from build123d import *

# Parameters (mm, degrees)
F0_R      = 7.65
F0_R_2    = 4.65
F1_DEPTH  = 20
F4_DEPTH  = 20.001
F6_R      = 0.775
F7_DEPTH  = 1.0786128078
F9_R      = 0.775
F10_DEPTH = 1.0463142634
F12_R     = 0.775
F13_DEPTH = 1.0463142634
F14_W     = 1
F14_H     = 5.2947397344
F15_DEPTH = 20
F16_R     = 0.835
F17_DEPTH = 20
F18_W     = 3.1734104046
F18_H     = 10
F19_DEPTH = 15.2846427429


with BuildPart() as f1:
    # F0 (on Top) → F1 (new body)
    with BuildSketch(Plane.XY):
        Circle(F0_R)
        Circle(F0_R_2, mode=Mode.SUBTRACT)
    extrude(amount=F1_DEPTH)

    # F2 (on face) → F4 (cut, through all)
    with BuildSketch(Plane.XY.offset(20)):
        with BuildLine():
            Line((-3.4395020739, 4.4824463726), (-4.0482635029, 5.2757997129))
            ThreePointArc((-4.0482635029, 5.2757997129), (-5.7590689352, 3.325), (-6.5931083281, 0.8679991783))
            Line((-6.5931083281, 0.8679991783), (-5.6016634668, 0.737472986))
            ThreePointArc((-5.6016634668, 0.737472986), (-4.8930435314, 2.825), (-3.4395020739, 4.4824463726))
        make_face()
        with BuildLine():
            Line((4.0482635029, 5.2757997129), (3.4395020739, 4.4824463726))
            ThreePointArc((3.4395020739, 4.4824463726), (4.8930435314, 2.825), (5.6016634668, 0.737472986))
            Line((5.6016634668, 0.737472986), (6.5931083281, 0.8679991783))
            ThreePointArc((6.5931083281, 0.8679991783), (5.7590689352, 3.325), (4.0482635029, 5.2757997129))
        make_face()
        with BuildLine():
            ThreePointArc((2.1621613929, -5.2199193587), (0, -5.65), (-2.1621613929, -5.2199193587))
            Line((-2.1621613929, -5.2199193587), (-2.5448448252, -6.1437988912))
            ThreePointArc((-2.5448448252, -6.1437988912), (0, -6.65), (2.5448448252, -6.1437988912))
            Line((2.5448448252, -6.1437988912), (2.1621613929, -5.2199193587))
        make_face()
    extrude(amount=-F4_DEPTH, mode=Mode.SUBTRACT)

    # F6 (on line) → F7 (cut, through all)
    with BuildSketch(Plane(origin=(-6.625094339, 3.825, 0), x_dir=(0.5, 0.8660254038, 0), z_dir=(0.8660254038, -0.5, 0))):
        with Locations((0, 15)):
            Circle(F6_R)
        with Locations((-0.2380277795, 5.0028332626)):
            Circle(F6_R)
    extrude(amount=F7_DEPTH, mode=Mode.SUBTRACT)

    # F9 (on line) → F10 (cut, through all)
    with BuildSketch(Plane.XZ.offset(7.65)):
        with Locations((0, 5)):
            Circle(F9_R)
        with Locations((0, 15)):
            Circle(F9_R)
    extrude(amount=-F10_DEPTH, mode=Mode.SUBTRACT)

    # F12 (on line) → F13 (cut, through all)
    with BuildSketch(Plane(origin=(6.625094339, 3.825, 0), x_dir=(-0.5, 0.8660254038, 0), z_dir=(0.8660254038, 0.5, 0))):
        with Locations((0, 5)):
            Circle(F12_R)
        with Locations((0, 15)):
            Circle(F12_R)
    extrude(amount=-F13_DEPTH, mode=Mode.SUBTRACT)

    # F14 (on face) → F15 (cut, through all)
    with BuildSketch(Plane(origin=(0, 0, 0), x_dir=(1, 0, 0), z_dir=(0, 0, -1))):
        with Locations((0, -6.6740161274)):
            Rectangle(F14_W, F14_H)
    extrude(amount=-F15_DEPTH, mode=Mode.SUBTRACT)

    # F16 (on face) → F17 (join, through all)
    with BuildSketch(Plane.XY.offset(20)):
        with BuildLine():
            ThreePointArc((-7.4765895954, -1.6196011924), (-7.65, 0), (-7.4765895954, 1.6196011924))
            ThreePointArc((-7.4765895954, 1.6196011924), (-10.65, 0), (-7.4765895954, -1.6196011924))
        make_face()
        with Locations((-8.65, 0)):
            Circle(F16_R, mode=Mode.SUBTRACT)
        with BuildLine():
            ThreePointArc((7.4765895954, -1.6196011924), (9.5591697286, -1.7814068611), (10.65, 0))
            ThreePointArc((10.65, 0), (9.5591697286, 1.7814068611), (7.4765895954, 1.6196011924))
            ThreePointArc((7.4765895954, 1.6196011924), (7.606523858, 0.8144291238), (7.65, 0))
            ThreePointArc((7.65, 0), (7.606523858, -0.8144291238), (7.4765895954, -1.6196011924))
        make_face()
        with Locations((8.65, 0)):
            Circle(F16_R, mode=Mode.SUBTRACT)
    extrude(amount=-F17_DEPTH)

    # F18 (on line) → F19 (cut, through all)
    with BuildSketch(Plane.XZ.offset(7.65)):
        with Locations((-9.0632947977, 10)):
            Rectangle(F18_W, F18_H)
        with Locations((9.0632947977, 10)):
            Rectangle(F18_W, F18_H)
    extrude(amount=-F19_DEPTH, mode=Mode.SUBTRACT)


solid = f1.part
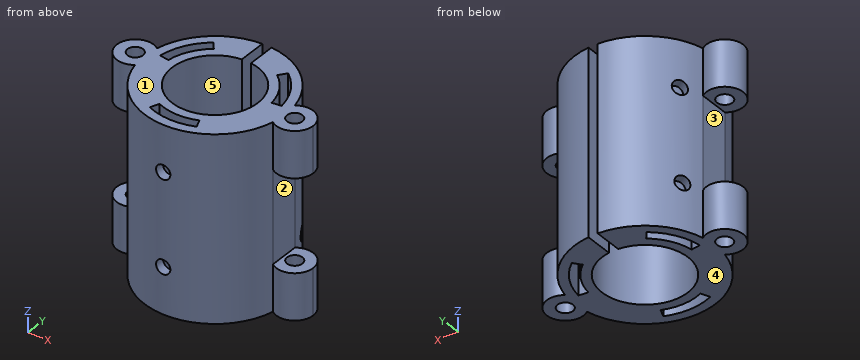
CAD build for the part. Positions are in the model's coordinates, mm. Face numbers are marked on the shaded views. A direction names the side the tool comes from. Round coordinates to 2 decimals unless told otherwise and drop trailing zeros. Write each loop counter-clockwise with the first axis right and the second up, starting at its lowest first coordinate (ties: lowest second). Pieces come first, ordered by that corner, then holes.
(1) Slice it at C-C, the plane z = 3.25. Count the separate pieces of the cut face and the enclosed holes in it, and give its area (3 significant figures).
(2) Slice it at B-B, the plane x = 8.65. Write the cut outline in (y, z) (3 decimals), and give its area (3 significant figures).
(3) Drop flat-ended pins along their axis: P1, Ø3, axis at x = -4.5, z = 10.5, coming from the +Y side; P2, Ø1.5, axis at x = -8.65, y = 0, coming from the +Z side; P3, Ø6, axis at y = 4.5, z = 16, coming from the -X side; P4, Ø2.5, axis at y = 0.5, z = 10.5, coming from the -X side. Give the stop position or say it passes through.
(4) Slice it at A-A, the plane z = 13.25. Write the cut outline in (x, y).
(5) Mould opens along Z. For the marked faces 3, 4 and 5 say: pulls with the +Z half, pulls with the -Z half, needs draft (parallel to the pull), parting line crosses it, or undercut.
(6) 3-axis set-ups, long thin cutter, end or side, ignore diameter. For the marked faces 1 and 2: which of +Z, -Z, +X, -X, +Y, -Y reach the whole face in a straight line?
(7) Probe line 1 along Z through (x, y) = (0, -6.95) (3 decimals); line 2 along Y through (x, z) = (-8.65, 2.9) (3 decimals); line 3 along X through (y, z) = (1, 8). List the from-to ranges inside material, lowest first.
(8) Slice it at D-D, the plane y = -3.5. Write the cut outline in (x, z), and give its area (3 significant figures).
From the geometry:
1. separate pieces: 1
1. enclosed holes: 5
1. area: 115 mm2
2. outline: (-2, 0) - (-0.835, 0) - (-0.835, 5) - (-2, 5) - close; (-2, 15) - (-0.835, 15) - (-0.835, 20) - (-2, 20) - close; (0.835, 0) - (2, 0) - (2, 5) - (0.835, 5) - close; (0.835, 15) - (2, 15) - (2, 20) - (0.835, 20) - close
2. area: 23.3 mm2
3. P1: stops at y = 7.04
3. P2: passes through
3. P3: stops at x = -9.97
3. P4: stops at x = -7.48
4. outline: (-7.48, -1.62) arc R7.65 ccw to (7.48, -1.62) - (7.48, 1.62) arc R7.65 ccw to (0.5, 7.63) - (0.5, 4.62) arc R4.65 cw (long way) to (-0.5, 4.62) - (-0.5, 7.63) arc R7.65 ccw to (-7.48, 1.62) - close; hole (-6.59, 0.87) - (-5.6, 0.74) arc R5.65 cw to (-3.44, 4.48) - (-4.05, 5.28) arc R6.65 ccw to start; hole (-2.54, -6.14) arc R6.65 ccw to (2.54, -6.14) - (2.16, -5.22) arc R5.65 cw to (-2.16, -5.22) - close; hole (3.44, 4.48) arc R5.65 cw to (5.6, 0.74) - (6.59, 0.87) arc R6.65 ccw to (4.05, 5.28) - close
5. face 3: undercut
5. face 4: pulls with the -Z half
5. face 5: needs draft
6. face 1: +Z, +X, -X, +Y, -Y
6. face 2: +X, +Y, -Y
7. line 1: z = 0 to 4.225, 5.775 to 14.225, 15.775 to 20
7. line 2: y = -2 to -0.835, 0.835 to 2
7. line 3: x = -7.48 to -6.57, -5.56 to -4.54, 4.54 to 5.56, 6.57 to 7.48
8. outline: (-6.8, 0) - (-3.06, 0) - (-3.06, 20) - (-6.8, 20) - close; (3.06, 0) - (6.8, 0) - (6.8, 20) - (3.06, 20) - close
8. area: 150 mm2
